Answer from the drawing. Dimensions are ordinates in mm from the lowest x, y and z of the part. A direction names the side the tool comes from. Coordinates: 2 decimals unless noted, no trailing zeros. Write each loop counter-clockwise with the first axis right and the second up, starting at its lowest first coordinate (ties: lowest second). Pieces come first, ordered by that corner, then holes.
(1) Section B-B on y = 4 is taken. Write down the section's boundary in (x, z), then the cut area to 3 significant figures.
(2) Given pin 1 (12.5 mm diameter, centred on x = 11.5, y = 14, fed in from -Z); pin 2 (12.5 mm diameter, centred on y = 35, z = 13.5, fed in from +X); pin 3 (20.5 mm diameter, centred on y = 19, z = 12, fed in from -X), each flat-ended and moving along its own axis, determine where each tip first touches the part or whether it passes through.
(3) Find the intervals of material crossed by probe 1 along Z at (x, y) = (48, 32); probe 2 along X at (y, z) = (45, 18.5), in increasing order.
(4) Section C-C on y = 30.5 is taken. Write down the section's boundary in (x, z), then the cut area to 3 significant figures.
(5) Section D-D on x = 9 is taken. Write down the section's boundary in (y, z), then the cut area to 3 significant figures.
(6) Which of the six approach directions +Z, -Z, +X, -X, +Y, -Y give full straight-line access (tool end or side, diameter ignored) to the marked faces 1, 2 and 3?
(7) Section A-A on x = 45 is taken. Write down the section's boundary in (y, z).
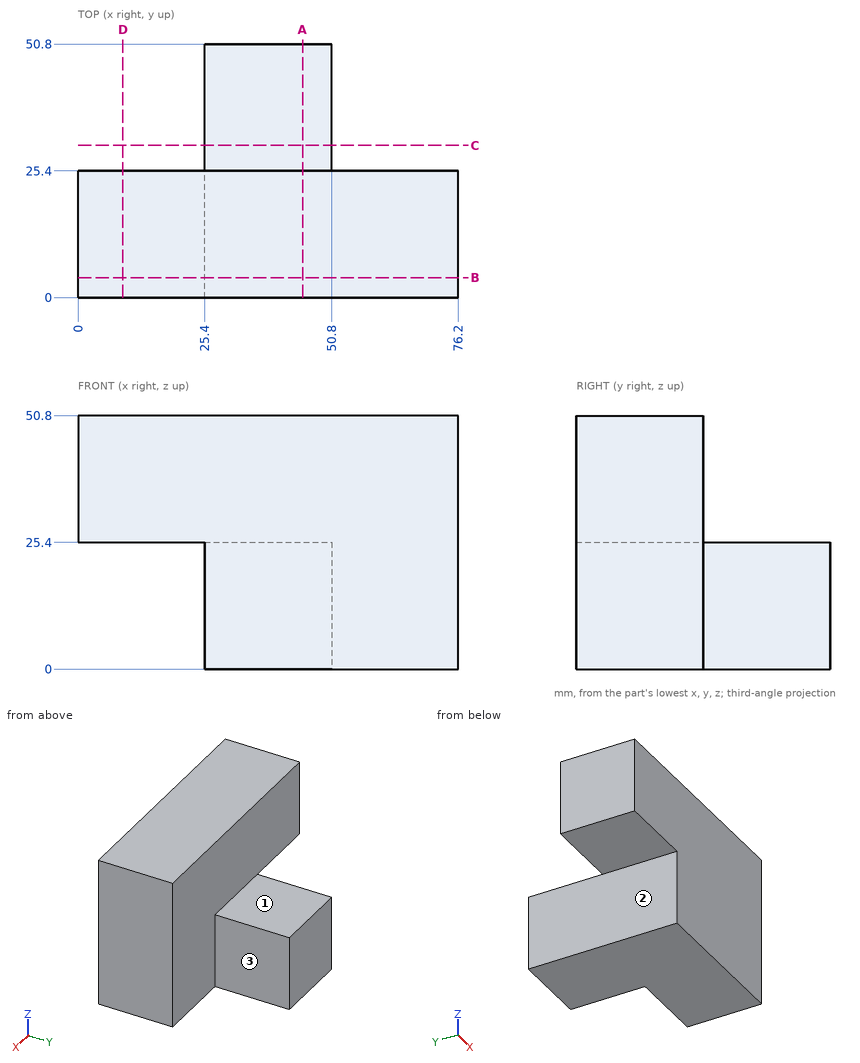
Response:
1. outline: (0, 25.4) - (25.4, 25.4) - (25.4, 0) - (76.2, 0) - (76.2, 50.8) - (0, 50.8) - close
1. area: 3,230 mm2
2. pin 1: stops at z = 25.4
2. pin 2: stops at x = 50.8
2. pin 3: stops at x = 25.4
3. probe 1: z = 0 to 25.4
3. probe 2: x = 25.4 to 50.8
4. outline: (25.4, 0) - (50.8, 0) - (50.8, 25.4) - (25.4, 25.4) - close
4. area: 645 mm2
5. outline: (0, 25.4) - (25.4, 25.4) - (25.4, 50.8) - (0, 50.8) - close
5. area: 645 mm2
6. face 1: +Z, +X, -X, +Y
6. face 2: -Z, -X, +Y, -Y
6. face 3: +Z, -Z, +X, +Y
7. outline: (0, 0) - (50.8, 0) - (50.8, 25.4) - (25.4, 25.4) - (25.4, 50.8) - (0, 50.8) - close
